Could you check a few things on this model? Use its own coordinates, in mm. Give positions to 0.01 mm unless a question says otherwise; leave off trailing zeros. One line per question, with ' | ' between items. Start each with the question number.
1. If we mould it in two halves opening along Z, with no side actions, what happens to faces 1 (the flat face through (4, 9, 15)), 2 (the flat face through (4, 9, -15)), 3 (the flat face through (4, -6, 0))? For each: released by +Z, released by -Z, zero draft, split by the parting line, or undercut.
2. I need wall thicknesses on probe 1 along Z at (x, y) = (88.5, -12); probe 2 along Z at (x, y) = (144.5, 3.75). Which ranges of each line are inside material? Lowest first, please. Write a range as from..to.
3. Imagine slicing it at A-A (x = 102). Give the number of separate pieces and of enclosed holes in the cut face, and give its area (3 significant figures).
4. For P1, Ø0.8, axis at x = -95, y = 14, coming from the -Z side; P2, Ø4, axis at x = 90.5, y = -0.5, coming from the -Z side; P3, Ø4, axis at x = 92, y = 1, coming from the +Z side, each with a flat end and sliding along its axis, tell me the tip position at first contact or that it passes through.
```python
from build123d import *

# Parameters (mm, degrees)
BR_EXTRUDE_DEPTH      = 275
BR_EXTRUDE_DEPTH_BACK = 275


with BuildPart() as part:
    # Sketch2 → BR_Extrude (new body, two sides)
    with BuildSketch(Plane(origin=(0, 0, 0), x_dir=(0, 0, -1), z_dir=(1, 0, 0))) as br_extrude_sk:
        with BuildLine():
            Line((-6, 4.196877708), (-10.053122292, 8.25))
            Line((-10.053122292, 8.25), (-12.8, 8.25))
            Line((-12.8, 8.25), (-12.800036742, 4.05))
            Line((-12.800036742, 4.05), (-14.5, 4.05))
            Line((-14.5, 4.05), (-14.5, 4.55))
            Line((-14.5, 4.55), (-15, 4.55))
            Line((-15, 4.55), (-15, 13))
            ThreePointArc((-15, 13), (-14.414213562, 14.414213562), (-13, 15))
            Line((-13, 15), (-4.55, 15))
            Line((-4.55, 15), (-4.55, 14.5))
            Line((-4.55, 14.5), (-4.05, 14.5))
            Line((-4.05, 14.5), (-4.05, 12.800036742))
            Line((-4.05, 12.800036742), (-8.25, 12.8))
            Line((-8.25, 12.8), (-8.25, 10.053122292))
            Line((-8.25, 10.053122292), (-4.196877708, 6))
            Line((-4.196877708, 6), (4.196877708, 6))
            Line((4.196877708, 6), (8.25, 10.053122292))
            Line((8.25, 10.053122292), (8.25, 12.8))
            Line((8.25, 12.8), (4.05, 12.800036742))
            Line((4.05, 12.800036742), (4.05, 14.5))
            Line((4.05, 14.5), (4.55, 14.5))
            Line((4.55, 14.5), (4.55, 15))
            Line((4.55, 15), (13, 15))
            ThreePointArc((13, 15), (14.414213562, 14.414213562), (15, 13))
            Line((15, 13), (15, 4.55))
            Line((15, 4.55), (14.5, 4.55))
            Line((14.5, 4.55), (14.5, 4.05))
            Line((14.5, 4.05), (12.800036742, 4.05))
            Line((12.800036742, 4.05), (12.8, 8.25))
            Line((12.8, 8.25), (10.053122292, 8.25))
            Line((10.053122292, 8.25), (6, 4.196877708))
            Line((6, 4.196877708), (6, -4.196877708))
            Line((6, -4.196877708), (10.053122292, -8.25))
            Line((10.053122292, -8.25), (12.8, -8.25))
            Line((12.8, -8.25), (12.800036742, -4.05))
            Line((12.800036742, -4.05), (14.5, -4.05))
            Line((14.5, -4.05), (14.5, -4.55))
            Line((14.5, -4.55), (15, -4.55))
            Line((15, -4.55), (15, -13))
            ThreePointArc((15, -13), (14.414213562, -14.414213562), (13, -15))
            Line((13, -15), (4.55, -15))
            Line((4.55, -15), (4.55, -14.5))
            Line((4.55, -14.5), (4.05, -14.5))
            Line((4.05, -14.5), (4.05, -12.800036742))
            Line((4.05, -12.800036742), (8.25, -12.8))
            Line((8.25, -12.8), (8.25, -10.053122292))
            Line((8.25, -10.053122292), (4.196877708, -6))
            Line((4.196877708, -6), (-4.196877708, -6))
            Line((-4.196877708, -6), (-8.25, -10.053122292))
            Line((-8.25, -10.053122292), (-8.25, -12.8))
            Line((-8.25, -12.8), (-4.05, -12.800036742))
            Line((-4.05, -12.800036742), (-4.05, -14.5))
            Line((-4.05, -14.5), (-4.55, -14.5))
            Line((-4.55, -14.5), (-4.55, -15))
            Line((-4.55, -15), (-13, -15))
            ThreePointArc((-13, -15), (-14.414213562, -14.414213562), (-15, -13))
            Line((-15, -13), (-15, -4.55))
            Line((-15, -4.55), (-14.5, -4.55))
            Line((-14.5, -4.55), (-14.5, -4.05))
            Line((-14.5, -4.05), (-12.800036742, -4.05))
            Line((-12.800036742, -4.05), (-12.8, -8.25))
            Line((-12.8, -8.25), (-10.053122292, -8.25))
            Line((-10.053122292, -8.25), (-6, -4.196877708))
            Line((-6, -4.196877708), (-6, 4.196877708))
        make_face()
        with BuildLine():
            Line((-13.85, -9.7), (-13.85, -12.85))
            ThreePointArc((-13.85, -12.85), (-13.557106781, -13.557106781), (-12.85, -13.85))
            Line((-12.85, -13.85), (-9.7, -13.85))
            Line((-9.7, -13.85), (-9.7, -9.7))
            Line((-9.7, -9.7), (-13.85, -9.7))
        make_face(mode=Mode.SUBTRACT)
        with BuildLine():
            Line((9.7, -13.85), (12.85, -13.85))
            ThreePointArc((12.85, -13.85), (13.557106781, -13.557106781), (13.85, -12.85))
            Line((13.85, -12.85), (13.85, -9.7))
            Line((13.85, -9.7), (9.7, -9.7))
            Line((9.7, -9.7), (9.7, -13.85))
        make_face(mode=Mode.SUBTRACT)
        with BuildLine():
            Line((13.85, 9.7), (13.85, 12.85))
            ThreePointArc((13.85, 12.85), (13.557106781, 13.557106781), (12.85, 13.85))
            Line((12.85, 13.85), (9.7, 13.85))
            Line((9.7, 13.85), (9.7, 9.7))
            Line((9.7, 9.7), (13.85, 9.7))
        make_face(mode=Mode.SUBTRACT)
        with BuildLine():
            Line((-9.7, 13.85), (-12.85, 13.85))
            ThreePointArc((-12.85, 13.85), (-13.557106781, 13.557106781), (-13.85, 12.85))
            Line((-13.85, 12.85), (-13.85, 9.7))
            Line((-13.85, 9.7), (-9.7, 9.7))
            Line((-9.7, 9.7), (-9.7, 13.85))
        make_face(mode=Mode.SUBTRACT)
        with BuildLine():
            Line((-3.272394192, -1.616767223), (-4.59052283, -3.187651763))
            Line((-4.59052283, -3.187651763), (-3.187651763, -4.59052283))
            Line((-3.187651763, -4.59052283), (-1.616767223, -3.272394192))
            ThreePointArc((-1.616767223, -3.272394192), (0, -3.65), (1.616767223, -3.272394192))
            Line((1.616767223, -3.272394192), (3.187651763, -4.59052283))
            Line((3.187651763, -4.59052283), (4.59052283, -3.187651763))
            Line((4.59052283, -3.187651763), (3.272394192, -1.616767223))
            ThreePointArc((3.272394192, -1.616767223), (3.65, 0), (3.272394192, 1.616767223))
            Line((3.272394192, 1.616767223), (4.59052283, 3.187651763))
            Line((4.59052283, 3.187651763), (3.187651763, 4.59052283))
            Line((3.187651763, 4.59052283), (1.616767223, 3.272394192))
            ThreePointArc((1.616767223, 3.272394192), (0, 3.65), (-1.616767223, 3.272394192))
            Line((-1.616767223, 3.272394192), (-3.187651763, 4.59052283))
            Line((-3.187651763, 4.59052283), (-4.59052283, 3.187651763))
            Line((-4.59052283, 3.187651763), (-3.272394192, 1.616767223))
            ThreePointArc((-3.272394192, 1.616767223), (-3.65, 0), (-3.272394192, -1.616767223))
        make_face(mode=Mode.SUBTRACT)
    extrude(amount=BR_EXTRUDE_DEPTH)
    extrude(br_extrude_sk.sketch, amount=-BR_EXTRUDE_DEPTH_BACK)


solid = part.part
```
Results found:
1) face 1: released by +Z | face 2: released by -Z | face 3: undercut
2) probe 1: z = -15..-13.85, -9.7..-8.25, 8.25..9.7, 13.85..15 | probe 2: z = -6..-4.03, -2.19..2.19, 4.03..6
3) separate pieces: 1 | enclosed holes: 5 | area: 314 mm2
4) P1: stops at z = -14.91 | P2: stops at z = -6 | P3: stops at z = 6
